Source: CAD feature listing. Evaluate the final solid. Frame: model axes, mm. A direction names the side the tool comes from. Give positions to 0.01 mm unless a question says otherwise; leave off trailing zeros. Loops run counter-clockwise (first coordinate to the right, second up) from the corner with the lowest first, then second, coordinate; pieces in that order, holes last. Notation, with made-up numbers: (-30.75, -9) - (-11.75, -9) arc R22 cw to (-11.75, 7) - close; hole circle Ø2 at (1.25, -12.75). An arc over 180 degrees is marked (long way). Put each result on its own line as item: value.
```python
from build123d import *

# Parameters (mm, degrees)
SKETCH1_R           = 1.5
SKETCH1_W           = 5
SKETCH1_H           = 5
BOSS_EXTRUDE1_DEPTH = 5
FILLET1_R           = 5


with BuildPart() as part:
    # Sketch1 → Boss-Extrude1 (new body)
    with BuildSketch(Plane.XY):
        Polygon((-65, -10), (-35, -10), (-35, 10), (35, 10), (35, -10), (65, -10), (65, 10), (20, 124), (20, 159), (-20, 159), (-20, 124), (-65, 10), align=None)
        with Locations((50, -2.5)):
            Circle(SKETCH1_R, mode=Mode.SUBTRACT)
        with Locations((-50, -2.5)):
            Circle(SKETCH1_R, mode=Mode.SUBTRACT)
        with Locations((0, 126.5)):
            Circle(SKETCH1_R, mode=Mode.SUBTRACT)
        with Locations((0, 151.5)):
            Circle(SKETCH1_R, mode=Mode.SUBTRACT)
        with Locations((42.5, -2.5)):
            Rectangle(SKETCH1_W, SKETCH1_H, mode=Mode.SUBTRACT)
        with Locations((57.5, -2.5)):
            Rectangle(SKETCH1_W, SKETCH1_H, mode=Mode.SUBTRACT)
        with Locations((-57.5, -2.5)):
            Rectangle(SKETCH1_W, SKETCH1_H, mode=Mode.SUBTRACT)
        with Locations((-42.5, -2.5)):
            Rectangle(SKETCH1_W, SKETCH1_H, mode=Mode.SUBTRACT)
        with Locations((-7.5, 126.5)):
            Rectangle(SKETCH1_W, SKETCH1_H, mode=Mode.SUBTRACT)
        with Locations((7.5, 126.5)):
            Rectangle(SKETCH1_W, SKETCH1_H, mode=Mode.SUBTRACT)
        with Locations((-7.5, 151.5)):
            Rectangle(SKETCH1_W, SKETCH1_H, mode=Mode.SUBTRACT)
        with Locations((7.5, 151.5)):
            Rectangle(SKETCH1_W, SKETCH1_H, mode=Mode.SUBTRACT)
    extrude(amount=BOSS_EXTRUDE1_DEPTH)

    # Fillet1
    fillet1_edges = [part.edges().sort_by_distance(p)[0] for p in [
        (-65, 10, 2.5),
        (-20, 124, 2.5),
        (-20, 159, 2.5),
        (20, 159, 2.5),
        (20, 124, 2.5),
        (65, 10, 2.5),
        (65, -10, 2.5),
        (35, -10, 2.5),
        (35, 10, 2.5),
        (-35, 10, 2.5),
        (-35, -10, 2.5),
        (-65, -10, 2.5),
    ]]
    fillet(fillet1_edges, radius=FILLET1_R)


solid = part.part
```
1) Access query for faces 1 (the flat face through (-8, 149, 2)), 2 (the flat face through (65, 2, 2)), 3 (the flat face through (-20, 140, 2)). Directions: +Z, -Z, +X, -X, +Y, -Y. A direction counts if a zero-diameter tool reaches every point of the face in a straight line with its end or side. Return the directions, or none.
Check result:
face 1: +Z, -Z
face 2: +Z, -Z, +X, +Y, -Y
face 3: +Z, -Z, -X, +Y
2) Section query C-C, the plane y = 145.5. Output: boundary loops of the cut face in (x, z), plus the area to 3 significant figures.
Check result:
outline: (-20, 0) - (20, 0) - (20, 5) - (-20, 5) - close
area: 200 mm²
3) Mould query, pull axis Y, two halves, no side actions, for faces 4 (the flat face through (-1, 57, 5)), 5 (the flat face through (50, -10, 2)), 6 (the flat face through (-10, 126, 2)). Classes: pulls with the +Y half, pulls with the -Y half, needs draft (parallel to the pull), parting line crosses it, or undercut.
Check result:
face 4: needs draft
face 5: pulls with the -Y half
face 6: undercut
4) Pin query (flat end, axial travel): P1, Ø1, axis at y = 19, z = 2, coming from the -X side; P2, Ø2, axis at x = 23, z = 1.5, coming from the -Y side; P3, Ø2.5, axis at y = 126.5, z = 1.5, coming from the +X side; P4, Ø2.5, axis at x = -50, y = -2.5, coming from the -Z side. Return the tip coordinate at first contact, or that it passes through.
Check result:
P1: x = -61.64
P2: y = 10
P3: x = 20
P4: through
5) Material intervals for line 1 along Y through (x, z) = (0, 3.4); line 2 along X through (y, z) = (4, 3.1); line 3 along X through (y, z) = (151.5, 3.75), sorted ascending. Write a range as [from, to].
Check result:
line 1: [10, 125], [128, 150], [153, 159]
line 2: [-65, -35], [35, 65]
line 3: [-20, -10], [-5, -1.5], [1.5, 5], [10, 20]
6) Section query B-B, the plane z = 3.55. State how many separate pieces and enclosed holes the cut face has, plus the area to 3 significant figures.
Check result:
separate pieces: 1
enclosed holes: 12
area: 12,000 mm²
7) Section query A-A, the plane y = 95.5. Output: boundary loops of the cut face in (x, z), plus the area to 4 significant figures.
Check result:
outline: (-31.25, 0) - (31.25, 0) - (31.25, 5) - (-31.25, 5) - close
area: 312.5 mm²
